Check sheet for the drawn part. Datum: minimum x, y, z corner. Units: mm. Give positions to 0.01 mm unless a question says otherwise; leave off trailing zeros. Loops run counter-clockwise (first coordinate to the right, second up) from the corner with the lowest first, then second, coordinate; pieces in that order, holes last.
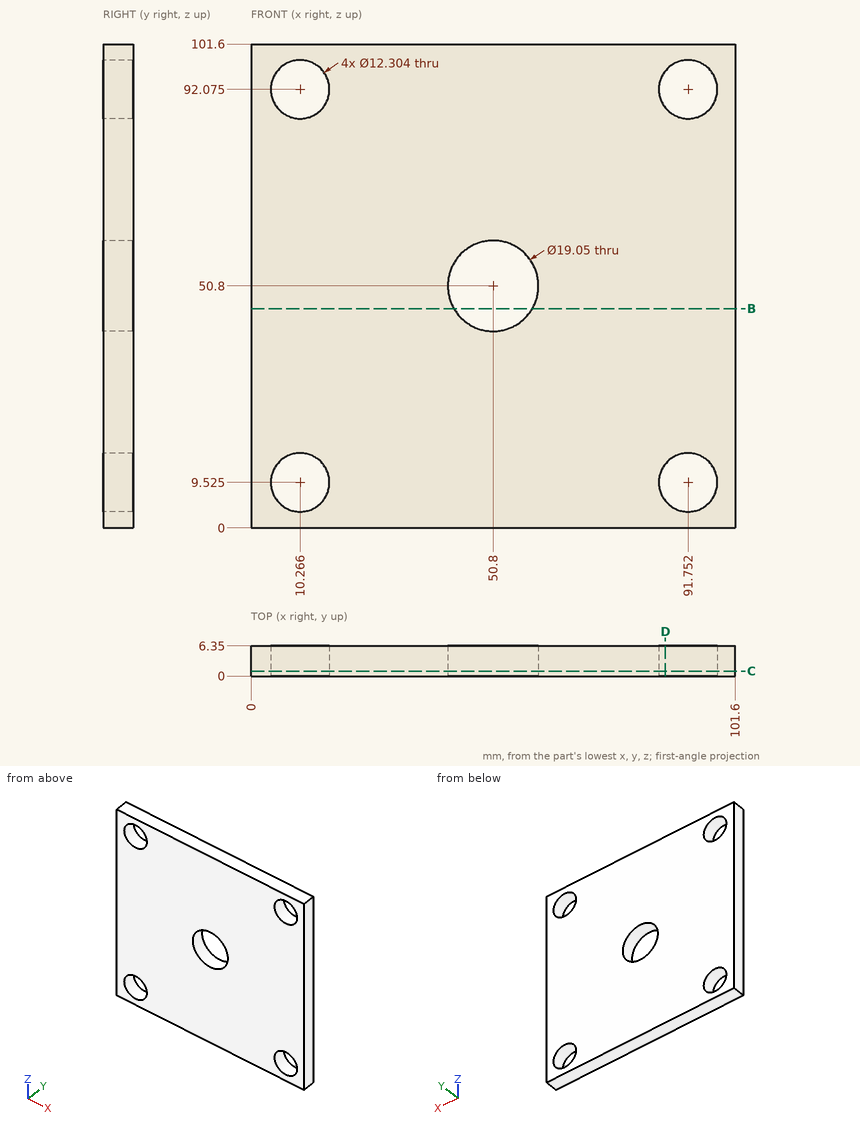
(1) Section check C-C on y = 1. Give the number of separate pieces and of enclosed holes in the cut face, plus the area to 3 significant figures.
(2) Section check D-D on x = 87. Record the boundary of the cut face in (y, z).
(3) Material ranges on line 1 (X direction, y = 2, z = 90) (1 decimal); line 2 (X direction, y = 4.5, z = 93.5); line 3 (Z direction, x = 12, y = 0.75), recorded low to high.
(4) Section check B-B on z = 46. Record the boundary of the cut face in (x, y).
Computed values:
1. separate pieces: 1
1. enclosed holes: 5
1. area: 9,560 mm2
2. outline: (0, 0) - (6.35, 0) - (6.35, 5.62) - (0, 5.62) - close; (0, 13.43) - (6.35, 13.43) - (6.35, 88.17) - (0, 88.17) - close; (0, 95.98) - (6.35, 95.98) - (6.35, 101.6) - (0, 101.6) - close
3. line 1: x = 0 to 4.5, 16.1 to 86, 97.5 to 101.6
3. line 2: x = 0 to 4.28, 16.25 to 85.77, 97.74 to 101.6
3. line 3: z = 0 to 3.62, 15.43 to 86.17, 97.98 to 101.6
4. outline: (0, 0) - (42.57, 0) - (42.57, 6.35) - (0, 6.35) - close; (59.03, 0) - (101.6, 0) - (101.6, 6.35) - (59.03, 6.35) - close
